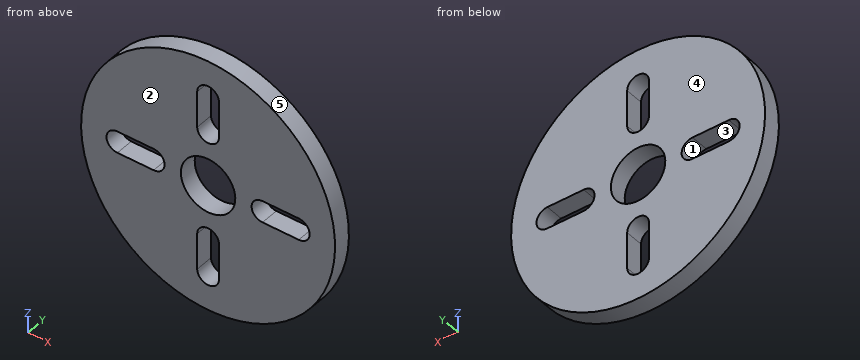
from build123d import *

# Parameters (mm, degrees)
SKETCH1_R           = 14
BOSS_EXTRUDE1_DEPTH = 2
SKETCH2_R           = 3
CUT_EXTRUDE1_DEPTH  = 20.899748742


with BuildPart() as part:
    # Sketch1 → Boss-Extrude1 (new body)
    with BuildSketch(Plane(origin=(0, 0, 0), x_dir=(1, 0, 0), z_dir=(0, 1, 0))):
        with Locations(Location((0, 0, 0), (0, 0, 270))):
            Circle(SKETCH1_R)
    extrude(amount=BOSS_EXTRUDE1_DEPTH)

    # Sketch2 → Cut-Extrude1 (cut, through all)
    with BuildSketch(Plane(origin=(0, 2, 0), x_dir=(1, 0, 0), z_dir=(0, 1, 0))):
        with Locations(Location((0, 0, 0), (0, 0, 270))):
            Circle(SKETCH2_R)
        with BuildLine():
            Line((1.2, 10), (1.2, 6))
            ThreePointArc((1.2, 6), (0, 4.8), (-1.2, 6))
            Line((-1.2, 6), (-1.2, 10))
            ThreePointArc((-1.2, 10), (0, 11.2), (1.2, 10))
        make_face()
        with BuildLine():
            Line((10, -1.2), (6, -1.2))
            ThreePointArc((6, -1.2), (4.8, 0), (6, 1.2))
            Line((6, 1.2), (10, 1.2))
            ThreePointArc((10, 1.2), (11.2, 0), (10, -1.2))
        make_face()
        with BuildLine():
            Line((-1.2, -10), (-1.2, -6))
            ThreePointArc((-1.2, -6), (0, -4.8), (1.2, -6))
            Line((1.2, -6), (1.2, -10))
            ThreePointArc((1.2, -10), (0, -11.2), (-1.2, -10))
        make_face()
        with BuildLine():
            Line((-10, 1.2), (-6, 1.2))
            ThreePointArc((-6, 1.2), (-4.8, 0), (-6, -1.2))
            Line((-6, -1.2), (-10, -1.2))
            ThreePointArc((-10, -1.2), (-11.2, 0), (-10, 1.2))
        make_face()
    extrude(amount=-CUT_EXTRUDE1_DEPTH, mode=Mode.SUBTRACT)


solid = part.part
Geometry: final body of the model. Coordinates: model frame, mm. Face numbers are marked on the shaded views. A direction names the side the tool comes from. Give positions to 0.01 mm unless a question says otherwise; leave off trailing zeros. Write each loop counter-clockwise with the first axis right and the second up, starting at its lowest first coordinate (ties: lowest second). Pieces come first, ordered by that corner, then holes. Notation, with made-up numbers: (72, -8.5) -> (121, -8.5) arc R22 ccw to (121, 10.5) -> close; hole circle Ø4 at (-26.75, 18.25). An arc over 180 degrees is marked (long way). Answer as a JSON object with one key per item and string values.
1. Cut plane C-C on y = 0.8. Output: boundary loops of the cut face in (x, z).
Ans:
{"outline": "circle Ø28 at (0, 0); hole (-10, -1.2) -> (-6, -1.2) arc R1.2 ccw to (-6, 1.2) -> (-10, 1.2) arc R1.2 ccw to start; hole circle Ø6 at (0, 0); hole (-1.2, -10) arc R1.2 ccw to (1.2, -10) -> (1.2, -6) arc R1.2 ccw to (-1.2, -6) -> close; hole (-1.2, 6) arc R1.2 ccw to (1.2, 6) -> (1.2, 10) arc R1.2 ccw to (-1.2, 10) -> close; hole (6, -1.2) -> (10, -1.2) arc R1.2 ccw to (10, 1.2) -> (6, 1.2) arc R1.2 ccw to start"}
2. Contact query for flat-ended pins moving along their axis: pin 1 (0.6 mm diameter, centred on y = 1, z = -8, fed in from +X); pin 2 (0.6 mm diameter, centred on x = 9, y = 1, fed in from -Z); pin 3 (1 mm diameter, centred on x = 7.5, y = 1, fed in from +Z). Output: stop coordinate, or through.
Ans:
{"pin 1": "stops at x = 11.69", "pin 2": "stops at z = -10.97", "pin 3": "stops at z = 12.12"}
3. Access query for the marked faces 1 and 2. Directions: +Z, -Z, +X, -X, +Y, -Y. A direction counts if a zero-diameter tool reaches every point of the face in a straight line with its end or side. Return the directions, or none.
Ans:
{"face 1": "+Y, -Y", "face 2": "+Z, -Z, +X, -X, -Y"}
4. Cut plane D-D on x = 10.5. Output: boundary loops of the cut face in (y, z), and give its area (3 significant figures).
Ans:
{"outline": "(0, -9.26) -> (2, -9.26) -> (2, -1.09) -> (0, -1.09) -> close; (0, 1.09) -> (2, 1.09) -> (2, 9.26) -> (0, 9.26) -> close", "area": "32.7 mm^2"}
5. Cut plane B-B on z = 0. Output: boundary loops of the cut face in (x, y), and give its area (3 significant figures).
Ans:
{"outline": "(-14, 0) -> (-11.2, 0) -> (-11.2, 2) -> (-14, 2) -> close; (-4.8, 0) -> (-3, 0) -> (-3, 2) -> (-4.8, 2) -> close; (3, 0) -> (4.8, 0) -> (4.8, 2) -> (3, 2) -> close; (11.2, 0) -> (14, 0) -> (14, 2) -> (11.2, 2) -> close", "area": "18.4 mm^2"}
6. Ray query, probe 1 along X at (y, z) = (1.55, 0); probe 2 along X at (y, z) = (1.25, -2); probe 3 along Z at (x, y) = (7, 1.7). Return the intervals inside material, ascending. Write a range as from..to.
Ans:
{"probe 1": "x = -14..-11.2, -4.8..-3, 3..4.8, 11.2..14", "probe 2": "x = -13.86..-2.24, 2.24..13.86", "probe 3": "z = -12.12..-1.2, 1.2..12.12"}
7. Cut plane A-A on x = 0. Output: boundary loops of the cut face in (y, z).
Ans:
{"outline": "(0, -14) -> (2, -14) -> (2, -11.2) -> (0, -11.2) -> close; (0, -4.8) -> (2, -4.8) -> (2, -3) -> (0, -3) -> close; (0, 3) -> (2, 3) -> (2, 4.8) -> (0, 4.8) -> close; (0, 11.2) -> (2, 11.2) -> (2, 14) -> (0, 14) -> close"}
8. Mould query, pull axis X, two halves, no side actions, for the marked faces 3, 4 and 5. Classes: pulls with the +X half, pulls with the -X half, needs draft (parallel to the pull), parting line crosses it, or undercut.
Ans:
{"face 3": "undercut", "face 4": "needs draft", "face 5": "parting line crosses it"}
